Model file for the job. Use its own axes, mm. Coordinates: 2 decimals unless noted, no trailing zeros. Order: outer loops, then holes, each group sorted by start corner. A loop starts at its lowest first (then second) coordinate and runs counter-clockwise, first axis right, second up. Notation, with made-up numbers: (74.5, -22.75) -> (127.5, -22.75) arc R38 ccw to (127.5, 15.25) -> close; hole circle Ø2 at (-26.75, 15.5). An arc over 180 degrees is marked (long way). Use CSV: the item, a comma, the result in double quotes. Start each with the question number.
(1) Probe L1, parallel to Y at x = -22, z = 1.05; L2, parallel to X at y = 12, z = 1.45; L3, parallel to X at y = 9.5, z = 1.1. List the from-to ranges inside material, lowest first.
(2) Cut at D-D on y = 9. Write the cut outline in (x, z), plus the area to 3 significant figures.
(3) Cut at A-A on x = -22. Write the cut outline in (y, z).
(4) Cut at C-C on x = 8.5. Write the cut outline in (y, z).
(5) Cut at B-B on y = 0.5. Write the cut outline in (x, z).
```python
from build123d import *

# Parameters (mm, degrees)
SZKIC1_R                    = 1.25
DODANIE_WYCI_GNI_CIE1_DEPTH = 2


with BuildPart() as part:
    # Szkic1 → Dodanie-wyciągnięcie1 (new body)
    with BuildSketch(Plane.XY):
        with BuildLine():
            Line((-27, -20), (27, -20))
            ThreePointArc((27, -20), (29.121320344, -19.121320344), (30, -17))
            Line((30, -17), (30, 17))
            ThreePointArc((30, 17), (29.121320344, 19.121320344), (27, 20))
            Line((27, 20), (-27, 20))
            ThreePointArc((-27, 20), (-29.121320344, 19.121320344), (-30, 17))
            Line((-30, 17), (-30, -17))
            ThreePointArc((-30, -17), (-29.121320344, -19.121320344), (-27, -20))
        make_face()
        with Locations((-22, 14.666666667)):
            Circle(SZKIC1_R, mode=Mode.SUBTRACT)
        with BuildLine():
            ThreePointArc((-25.462131621, -15.720072586), (-22, -15.916666667), (-18.537868379, -15.720072586))
            ThreePointArc((-18.537868379, -15.720072586), (-17.437407577, -14.336603749), (-18.820876413, -13.236142947))
            ThreePointArc((-18.820876413, -13.236142947), (-22, -13.416666667), (-25.179123587, -13.236142947))
            ThreePointArc((-25.179123587, -13.236142947), (-26.562592423, -14.336603749), (-25.462131621, -15.720072586))
        make_face(mode=Mode.SUBTRACT)
        with BuildLine():
            ThreePointArc((26.294998597, 4.920914996), (27.087801786, 10.450711145), (27.249518026, 16.034708834))
            ThreePointArc((27.249518026, 16.034708834), (25.965291166, 17.249518026), (24.750481974, 15.965291166))
            ThreePointArc((24.750481974, 15.965291166), (24.596971596, 10.664638616), (23.8443971, 5.415437293))
            ThreePointArc((23.8443971, 5.415437293), (24.8224367, 3.942875396), (26.294998597, 4.920914996))
        make_face(mode=Mode.SUBTRACT)
        with BuildLine():
            ThreePointArc((21.193691844, -16.735032503), (24.470809822, -11.643513117), (27.150485656, -6.213742466))
            ThreePointArc((27.150485656, -6.213742466), (26.488756334, -4.574500475), (24.849514344, -5.236229797))
            ThreePointArc((24.849514344, -5.236229797), (22.295287061, -10.411806693), (19.171586782, -15.264967497))
            ThreePointArc((19.171586782, -15.264967497), (19.44760681, -17.011052531), (21.193691844, -16.735032503))
        make_face(mode=Mode.SUBTRACT)
        with BuildLine():
            ThreePointArc((6.601254034, -9.49476923), (9.152553238, -6.101702158), (11.303346225, -2.441630943))
            ThreePointArc((11.303346225, -2.441630943), (6.545275723, 12.369201751), (-8.265556972, 7.611131249))
            ThreePointArc((-8.265556972, 7.611131249), (-9.152553238, 6.101702158), (-10.204719988, 4.702386724))
            ThreePointArc((-10.204719988, 4.702386724), (-8.900310954, -10.799178264), (6.601254034, -9.49476923))
        make_face(mode=Mode.SUBTRACT)
    extrude(amount=DODANIE_WYCI_GNI_CIE1_DEPTH)


solid = part.part
```
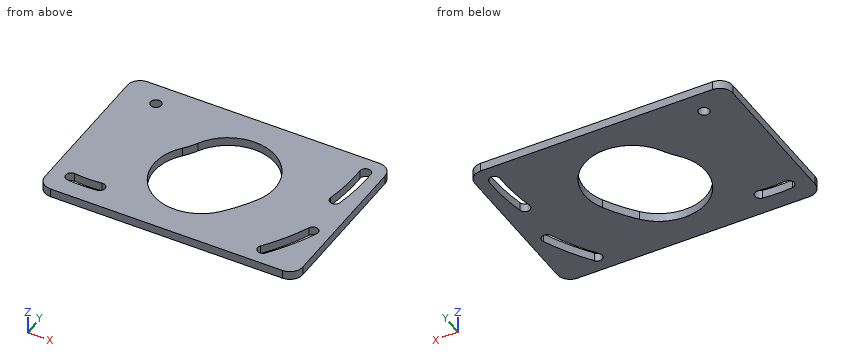
Outcome:
1,L1,"-20 to -15.92, -13.42 to 13.42, 15.92 to 20"
1,L2,"-30 to -4.17, 7.21 to 24.69, 27.2 to 30"
1,L3,"-30 to -7.04, 10.07 to 24.48, 27 to 30"
2,outline,"(-30, 0) -> (-7.42, 0) -> (-7.42, 2) -> (-30, 2) -> close; (10.45, 0) -> (24.42, 0) -> (24.42, 2) -> (10.45, 2) -> close; (26.94, 0) -> (30, 0) -> (30, 2) -> (26.94, 2) -> close"
2,area,"79.2 mm2"
3,outline,"(-20, 0) -> (-15.92, 0) -> (-15.92, 2) -> (-20, 2) -> close; (-13.42, 0) -> (13.42, 0) -> (13.42, 2) -> (-13.42, 2) -> close; (15.92, 0) -> (20, 0) -> (20, 2) -> (15.92, 2) -> close"
4,outline,"(-20, 0) -> (-7.05, 0) -> (-7.05, 2) -> (-20, 2) -> close; (11.09, 0) -> (20, 0) -> (20, 2) -> (11.09, 2) -> close"
5,outline,"(-30, 0) -> (-12.41, 0) -> (-12.41, 2) -> (-30, 2) -> close; (12.32, 0) -> (30, 0) -> (30, 2) -> (12.32, 2) -> close"
